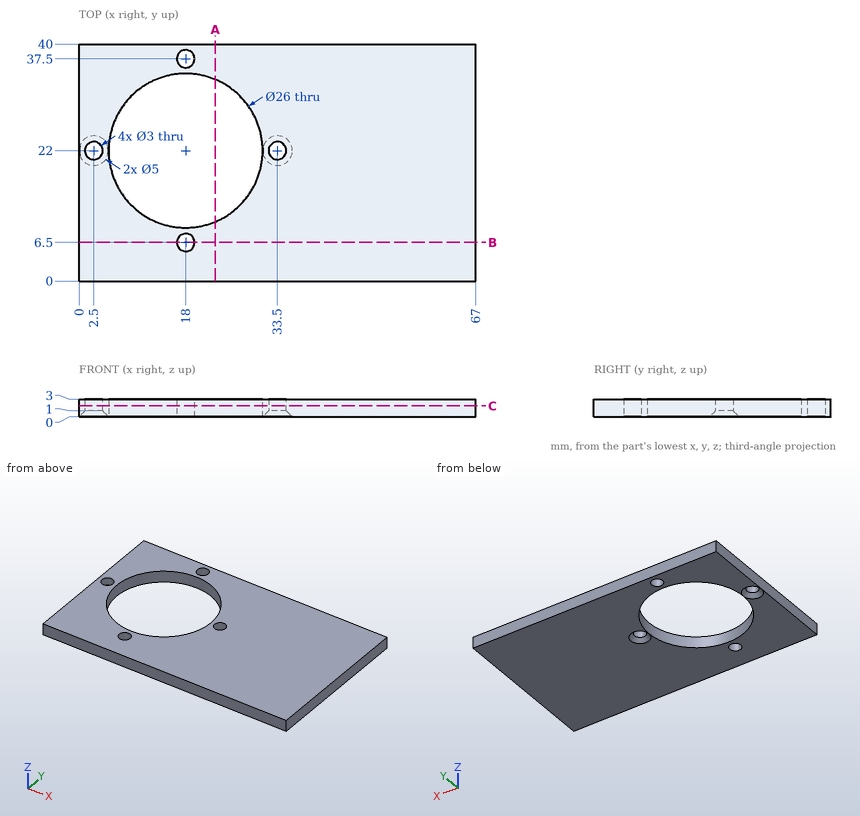
Answer from the drawing. Dimensions are ordinates in mm from the lowest x, y and z of the part. Coordinates: 2 decimals unless noted, no trailing zeros. Order: outer loops, then holes, each group sorted by start corner. A loop starts at its lowest first (then second) coordinate and runs counter-clockwise, first axis right, second up. Notation, with made-up numbers: (-39.75, -36.75) - (-15.75, -36.75) arc R20 cw to (-15.75, -30.75) - close; hole circle Ø2 at (65.5, 81). An arc over 180 degrees is marked (long way). Answer as a JSON object with one key per item and string values. Group by question number.
Item 1: Consider probe 1 along Y at (x, z) = (18, 1.6); probe 2 along X at (y, z) = (21.5, 1.6); probe 3 along Y at (x, z) = (3.5, 2.5). Determine where each line is inside the solid, lowest interval first. Write a range as from..to.
Item 2: Section A-A (x = 23) is taken. Give the vertices of the cut face in (y, z).
Item 3: Flat-ended cylindrical pins translate along their axes: P1, Ø1.5, axis at y = 22, z = 2, coming from the -X side; P2, Ø2.5, axis at x = 2.5, y = 22, coming from the +Z side. Find the tip coordinate at first contact, or state that the pin passes through.
Item 4: Section C-C (z = 1.85) is taken. Give the vertices of the cut face in (x, y), plus the area to 3 significant figures.
Item 5: Section B-B (y = 6.5) is taken. Give the vertices of the cut face in (x, z).
Results are:
{
 "1": {"probe 1": "y = 0..5, 8..9, 35..36, 39..40", "probe 2": "x = 0..1.09, 3.91..5.01, 30.99..32.09, 34.91..67", "probe 3": "y = 0..20.88, 23.12..40"},
 "2": {"outline": "(0, 0) - (10, 0) - (10, 3) - (0, 3) - close; (34, 0) - (40, 0) - (40, 3) - (34, 3) - close"},
 "3": {"P1": "stops at x = 0", "P2": "passes through"},
 "4": {"outline": "(0, 0) - (67, 0) - (67, 40) - (0, 40) - close; hole circle Ø3 at (2.5, 22); hole circle Ø26 at (18, 22); hole circle Ø3 at (18, 6.5); hole circle Ø3 at (18, 37.5); hole circle Ø3 at (33.5, 22)", "area": "2,120 mm^2"},
 "5": {"outline": "(0, 0) - (16.5, 0) - (16.5, 3) - (0, 3) - close; (19.5, 0) - (67, 0) - (67, 3) - (19.5, 3) - close"}
}
